from build123d import *

# Parameters (mm, degrees)
RESSALTO_EXTRUS_O1_DEPTH = 2
ESBO_O2_R                = 0.25
CORTE_EXTRUS_O2_DEPTH    = 2


with BuildPart() as part:
    # Esboço1 → Ressalto-extrusão1 (new body)
    with BuildSketch(Plane.XY):
        with BuildLine():
            Line((104.678372413, -2.590763748), (101.678372413, -2.590763748))
            Line((101.678372413, -2.590763748), (101.678372413, -7.720763748))
            ThreePointArc((101.678372413, -7.720763748), (96.678372413, -12.720763748), (91.678372413, -7.720763748))
            Line((91.678372413, -7.720763748), (91.678372413, -2.590763748))
            Line((91.678372413, -2.590763748), (88.678372413, -2.590763748))
            Line((88.678372413, -2.590763748), (88.678372413, -2.770763748))
            Line((88.678372413, -2.770763748), (91.528372413, -2.770763748))
            Line((91.528372413, -2.770763748), (91.528372413, -7.720763748))
            ThreePointArc((91.528372413, -7.720763748), (96.678372413, -12.870763748), (101.828372413, -7.720763748))
            Line((101.828372413, -7.720763748), (101.828372413, -2.770763748))
            Line((101.828372413, -2.770763748), (104.678372413, -2.770763748))
            Line((104.678372413, -2.770763748), (104.678372413, -2.590763748))
        make_face()
    extrude(amount=RESSALTO_EXTRUS_O1_DEPTH)

    # Esboço2 → Corte-extrusão2 (cut)
    with BuildSketch(Plane.XZ.offset(2.770763748)):
        with Locations(Location((90.103372413, 1, 0), (0, 0, 270))):
            Circle(ESBO_O2_R)
        with Locations(Location((103.253372413, 1, 0), (0, 0, 270))):
            Circle(ESBO_O2_R)
    extrude(amount=-CORTE_EXTRUS_O2_DEPTH, mode=Mode.SUBTRACT)


solid = part.part
Verification items for the finished model (mm, model axes). A direction names the side the tool comes from. Round coordinates to 2 decimals unless told otherwise and drop trailing zeros. Loops run counter-clockwise (first coordinate to the right, second up) from the corner with the lowest first, then second, coordinate; pieces in that order, holes last. Notation, with made-up numbers: (36, -1.5) - (43, -1.5) arc R14 ccw to (43, 13.5) - close; hole circle Ø8 at (10, 62). An arc over 180 degrees is marked (long way). Answer in a Markdown table with one row per item. Add a question column.
Q1. Section check C-C on x = 102.75. Enter the section's corners in (y, z), plus the area to 3 significant figures.
Q2. Section check A-A on z = 1. Enter the section's corners in (x, y).
Q3. Section check D-D on y = -12. Enter the section's corners in (x, z).
Q4. Section check B-B on y = -9.5. Enter the section's corners in (x, z), plus the area to 3 significant figures.
Q5. Gauge pin test, flat ends, axial feed: pin 1 (1 mm diameter, centred on x = 103, z = 1.5, fed in from -Y); pin 2 (1 mm diameter, centred on y = -4, z = 0.5, fed in from +X); pin 3 (1 mm diameter, centred on y = -5, z = 1, fed in from -X). Record the tip position at first contact, or that the pin passes through.
Q6. Tool access check on faces 1 (the face through (89.77, -2.771, 0.76)), 2 (the face through (91, -2.591, 1)). Record the directions out of +Z, -Z, +X, -X, +Y, -Y that give a thin tool (end or side, any length) a straight path to the whole face; none if there is none.
Q7. Release check for a two-part mould opening along X. For faces 3 (the face through (104, -2.771, 1)), 4 (the face through (101.678, -5, 1)), 5 (the face through (91.528, -5, 1)), 6 (the face through (96.57, -12.87, 0.99)) record: pulls with the +X half, pulls with the -X half, needs draft (parallel to the pull), parting line crosses it, or undercut.
Q8. Material ranges on line 1 (X direction, y = -2.7, z = 1); line 2 (Y direction, x = 104.25, z = 1); line 3 (X direction, y = -11.75, z = 1.3), recorded low to high.
Found:
| question | item | result |
|---|---|---|
| 1 | outline | (-2.77, 0) - (-2.59, 0) - (-2.59, 2) - (-2.77, 2) - close |
| 1 | area | 0.360 mm² |
| 2 | outline | (88.68, -2.77) - (89.85, -2.77) - (89.85, -2.59) - (88.68, -2.59) - close; (90.35, -2.77) - (91.53, -2.77) - (91.53, -7.72) arc R5.15 ccw to (101.83, -7.72) - (101.83, -2.77) - (103, -2.77) - (103, -2.59) - (101.68, -2.59) - (101.68, -7.72) arc R5 cw to (91.68, -7.72) - (91.68, -2.59) - (90.35, -2.59) - close; (103.5, -2.77) - (104.68, -2.77) - (104.68, -2.59) - (103.5, -2.59) - close |
| 3 | outline | (93.81, 0) - (94.09, 0) - (94.09, 2) - (93.81, 2) - close; (99.26, 0) - (99.54, 0) - (99.54, 2) - (99.26, 2) - close |
| 4 | outline | (91.85, 0) - (92.01, 0) - (92.01, 2) - (91.85, 2) - close; (101.35, 0) - (101.51, 0) - (101.51, 2) - (101.35, 2) - close |
| 4 | area | 0.641 mm² |
| 5 | pin 1 | stops at y = -2.77 |
| 5 | pin 2 | stops at x = 101.83 |
| 5 | pin 3 | stops at x = 91.53 |
| 6 | face 1 | +Z, -Z, -X, -Y |
| 6 | face 2 | +Z, -Z, +X, -X, +Y |
| 7 | face 3 | needs draft |
| 7 | face 4 | undercut |
| 7 | face 5 | pulls with the -X half |
| 7 | face 6 | parting line crosses it |
| 8 | line 1 | x = 88.68 to 89.85, 90.35 to 91.68, 101.68 to 103, 103.5 to 104.68 |
| 8 | line 2 | y = -2.77 to -2.59 |
| 8 | line 3 | x = 93.47 to 93.72, 99.64 to 99.89 |
